from build123d import *

# Parameters (mm, degrees)
SKETCH1_W           = 50.8
SKETCH1_H           = 22.225
BOSS_EXTRUDE1_DEPTH = 12.7
SKETCH2_R           = 2.2
CUT_EXTRUDE1_DEPTH  = 57.884801353
SKETCH4_R           = 1.7525
CUT_EXTRUDE3_DEPTH  = 3.4
CUT_EXTRUDE4_START  = -3.4
SKETCH4_3_R         = 1.7525
CUT_EXTRUDE4_DEPTH  = 1
CUT_EXTRUDE5_REACH  = 57.198
SKETCH4_4_R         = 1.7525
FILLET1_R           = 3
FILLET2_R           = 2
FILLET3_R           = 2


with BuildPart() as part:
    # Sketch1 → Boss-Extrude1 (new body)
    with BuildSketch(Plane(origin=(0, 0, 0), x_dir=(1, 0, 0), z_dir=(0, 1, 0))):
        with Locations((-25.4, -11.1125)):
            Rectangle(SKETCH1_W, SKETCH1_H)
    extrude(amount=BOSS_EXTRUDE1_DEPTH)

    # Sketch2 → Cut-Extrude1 (cut, through all)
    with BuildSketch(Plane.ZY.offset(50.8)):
        with Locations((4.7625, 6.35)):
            Circle(SKETCH2_R)
    extrude(amount=-CUT_EXTRUDE1_DEPTH, mode=Mode.SUBTRACT)

    # Sketch4 → Cut-Extrude3 (cut)
    # profile 1 of 9: a face of its own
    with BuildSketch(Plane.XY.offset(17.4625)):
        Polygon((-40.3, 12.7), (-40.3, 8.746003617), (-44.45, 11.142007234), (-48.6, 8.746003617), (-48.6, 12.7), align=None)
    # profile 2 of 9: a face of its own
    with BuildSketch(Plane.XY.offset(17.4625)):
        Polygon((-48.6, 8.746003617), (-48.6, 3.953996383), (-44.45, 1.557992766), (-40.3, 3.953996383), (-40.3, 8.746003617), (-44.45, 11.142007234), align=None)
        with Locations((-44.45, 6.35)):
            Circle(SKETCH4_R, mode=Mode.SUBTRACT)
    # profile 3 of 9: a face of its own
    with BuildSketch(Plane.XY.offset(17.4625)):
        Polygon((-35.9, 12.7), (-27.6, 12.7), (-27.6, 8.746003617), (-27.6, 3.953996383), (-31.75, 1.557992766), (-35.9, 3.953996383), (-35.9, 8.746003617), align=None)
        with Locations((-31.75, 6.35)):
            Circle(SKETCH4_R, mode=Mode.SUBTRACT)
    # profile 4 of 9: a face of its own
    with BuildSketch(Plane.XY.offset(17.4625)):
        with Locations((-31.75, 6.35)):
            Circle(SKETCH4_R)
    # profile 5 of 9: a face of its own
    with BuildSketch(Plane.XY.offset(17.4625)):
        with Locations((-44.45, 6.35)):
            Circle(SKETCH4_R)
    # profile 6 of 9: a face of its own
    with BuildSketch(Plane.XY.offset(17.4625)):
        Polygon((-23.2, 12.7), (-14.9, 12.7), (-14.9, 8.746003617), (-14.9, 3.953996383), (-19.05, 1.557992766), (-23.2, 3.953996383), (-23.2, 8.746003617), align=None)
        with Locations((-19.05, 6.35)):
            Circle(SKETCH4_R, mode=Mode.SUBTRACT)
    # profile 7 of 9: a face of its own
    with BuildSketch(Plane.XY.offset(17.4625)):
        with Locations((-19.05, 6.35)):
            Circle(SKETCH4_R)
    # profile 8 of 9: a face of its own
    with BuildSketch(Plane.XY.offset(17.4625)):
        Polygon((-10.5, 12.7), (-2.2, 12.7), (-2.2, 8.746003617), (-2.2, 3.953996383), (-6.35, 1.557992766), (-10.5, 3.953996383), (-10.5, 8.746003617), align=None)
        with Locations((-6.35, 6.35)):
            Circle(SKETCH4_R, mode=Mode.SUBTRACT)
    # profile 9 of 9: a face of its own
    with BuildSketch(Plane.XY.offset(17.4625)):
        with Locations((-6.35, 6.35)):
            Circle(SKETCH4_R)
    extrude(amount=-CUT_EXTRUDE3_DEPTH, mode=Mode.SUBTRACT)

    # Sketch4<3> → Cut-Extrude4 (cut)
    with BuildSketch(Plane.XY.offset(17.4625).offset(CUT_EXTRUDE4_START)):
        with Locations((-44.45, 6.35)):
            Circle(SKETCH4_3_R)
        with Locations((-31.75, 6.35)):
            Circle(SKETCH4_3_R)
        with Locations((-19.05, 6.35)):
            Circle(SKETCH4_3_R)
        with Locations((-6.35, 6.35)):
            Circle(SKETCH4_3_R)
    extrude(amount=-CUT_EXTRUDE4_DEPTH, mode=Mode.SUBTRACT)

    # Sketch4<4> → Cut-Extrude5 (cut, up to next)
    with BuildSketch(Plane.XY.offset(17.4625), mode=Mode.PRIVATE) as cut_extrude5_sk1:
        with Locations((-44.45, 6.35)):
            Circle(SKETCH4_4_R)
    cut_extrude5_tool1 = extrude(cut_extrude5_sk1.sketch, amount=CUT_EXTRUDE5_REACH, mode=Mode.PRIVATE) & part.part
    # Sketch4<4> → Cut-Extrude5 (cut, up to next)
    with BuildSketch(Plane.XY.offset(17.4625), mode=Mode.PRIVATE) as cut_extrude5_sk2:
        with Locations((-31.75, 6.35)):
            Circle(SKETCH4_4_R)
    cut_extrude5_tool2 = extrude(cut_extrude5_sk2.sketch, amount=CUT_EXTRUDE5_REACH, mode=Mode.PRIVATE) & part.part
    # Sketch4<4> → Cut-Extrude5 (cut, up to next)
    with BuildSketch(Plane.XY.offset(17.4625), mode=Mode.PRIVATE) as cut_extrude5_sk3:
        with Locations((-19.05, 6.35)):
            Circle(SKETCH4_4_R)
    cut_extrude5_tool3 = extrude(cut_extrude5_sk3.sketch, amount=CUT_EXTRUDE5_REACH, mode=Mode.PRIVATE) & part.part
    # Sketch4<4> → Cut-Extrude5 (cut, up to next)
    with BuildSketch(Plane.XY.offset(17.4625), mode=Mode.PRIVATE) as cut_extrude5_sk4:
        with Locations((-6.35, 6.35)):
            Circle(SKETCH4_4_R)
    cut_extrude5_tool4 = extrude(cut_extrude5_sk4.sketch, amount=CUT_EXTRUDE5_REACH, mode=Mode.PRIVATE) & part.part
    add(cut_extrude5_tool1.solids().sort_by_distance((-44.45, 6.35, 17.4625))[0], mode=Mode.SUBTRACT)
    add(cut_extrude5_tool2.solids().sort_by_distance((-31.75, 6.35, 17.4625))[0], mode=Mode.SUBTRACT)
    add(cut_extrude5_tool3.solids().sort_by_distance((-19.05, 6.35, 17.4625))[0], mode=Mode.SUBTRACT)
    add(cut_extrude5_tool4.solids().sort_by_distance((-6.35, 6.35, 17.4625))[0], mode=Mode.SUBTRACT)

    # Fillet1
    fillet1_edges = [part.edges().sort_by_distance(p)[0] for p in [
        (-25.4, 0, 0),
        (-25.4, 12.7, 0),
    ]]
    fillet(fillet1_edges, radius=FILLET1_R)

    # Fillet2
    fillet2_edges = [part.edges().sort_by_distance(p)[0] for p in [
        (-25.4, 12.7, 22.225),
        (-25.4, 0, 22.225),
    ]]
    fillet(fillet2_edges, radius=FILLET2_R)

    # Fillet3
    fillet3_edges = [part.edges().sort_by_distance(p)[0] for p in [
        (-50.8, 6.35, 0),
        (0, 6.35, 0),
        (-50.8, 0, 11.6125),
        (-50.8, 12.7, 11.6125),
        (-50.8, 11.821320344, 0.878679656),
        (-50.8, 0.878679656, 0.878679656),
        (0, 11.821320344, 0.878679656),
        (0, 0.878679656, 0.878679656),
        (0, 6.35, 22.225),
        (-50.8, 6.35, 22.225),
        (0, 0, 11.6125),
        (0, 12.7, 11.6125),
        (0, 12.114213562, 21.639213562),
        (0, 0.585786438, 21.639213562),
        (-50.8, 12.114213562, 21.639213562),
        (-50.8, 0.585786438, 21.639213562),
    ]]
    fillet(fillet3_edges, radius=FILLET3_R)


solid = part.part
Geometry: final body of the model. Coordinates: model frame, mm. A direction names the side the tool comes from. Round coordinates to 2 decimals unless told otherwise and drop trailing zeros. Loops run counter-clockwise (first coordinate to the right, second up) from the corner with the lowest first, then second, coordinate; pieces in that order, holes last. Notation, with made-up numbers: M 29,-14.5 L 42,-14.5 A27 cw 42,11.5 Z; hole C -24.75,-12.75 d4. An arc over 180 degrees is marked long. One line per question, with ' | ' between items.
(1) Pull-direction query (X, two-part tool) for faces 1 (the cylindrical face through (-50.23, 6.289, 21.624)), 2 (the cylindrical face through (-25.76, 5.01, 3.02)), 3 (the cylindrical face through (-20.44, 5.28, 13.57)); classes: +X half, -X half, draft (parallel to the pull), parting line (faces both ways), or undercut.
Check result:
face 1: -X half | face 2: draft | face 3: undercut
(2) Cut plane C-C on z = 3.75. Return the cut outline in (x, y), plus the area to 3 significant figures.
Check result:
outline: M -50.8,2 A2 ccw -48.8,0 L -2,0 A2 ccw 0,2 L 0,4.4 L -50.8,4.4 Z; M -50.8,8.3 L 0,8.3 L 0,10.7 A2 ccw -2,12.7 L -48.8,12.7 A2 ccw -50.8,10.7 Z | area: 443 mm2
(3) Cut plane A-A on z = 19. Give the number of separate pieces and of enclosed holes in the cut face, plus the area to 3 significant figures.
Check result:
separate pieces: 1 | enclosed holes: 4 | area: 603 mm2
(4) Contact query for a flat-ended pin moving along its axis: P1, Ø3, axis at x = -31.75, y = 6.35, coming from the +Z side. Output: stop coordinate, or through.
Check result:
P1: stops at z = 13.06
(5) Material intervals for line 1 along X through (y, z) = (6.35, 19.15); line 2 along Z through (x, y) = (-10, 6.25) (1 decimal); line 3 along Z through (x, y) = (-35, 3.5) (1 decimal), sorted ascending. Write a range as from..to.
Check result:
line 1: x = -50.8..-46.2, -42.7..-33.5, -30..-20.8, -17.3..-8.1, -4.6..0 | line 2: z = 0..2.6, 7..14.1, 17.5..22.2 | line 3: z = 0..14.1, 17.5..22.2
(6) Access query for faces 4 (the flat face through (-6.3, 8.4, 17.462)), 5 (the cylindrical face through (-42.78, 6.88, 13.57)), 6 (the cylindrical face through (-50.23, 6.4, 0.6)). Directions: +Z, -Z, +X, -X, +Y, -Y. A direction counts if a zero-diameter tool reaches every point of the face in a straight line with its end or side. Return the directions, or none.
Check result:
face 4: +Y | face 5: +Z | face 6: -Z, -X, +Y, -Y
